Part model, mm, in its own coordinate system. A direction names the side the tool comes from. Coordinates: 2 decimals unless noted, no trailing zeros. Loops run counter-clockwise (first coordinate to the right, second up) from the corner with the lowest first, then second, coordinate; pieces in that order, holes last.
Autodesk Inventor part; units mm, degrees
ref_plane "YZ Plane" through (0, 0, 0) normal (1, 0, 0) x (0, 1, 0)
ref_plane "XZ Plane" through (0, 0, 0) normal (0, 1, 0) x (-1, 0, 0)
ref_plane "XY Plane" through (0, 0, 0) normal (0, 0, 1) x (1, 0, 0)
sketch "Sketch1" plane through (0, 0, 0) normal (0, 1, 0) x (-1, 0, 0)
  line L0 (82, 45) -> (-82, 45)
  line L1 (-90, 37) -> (-90, -37)
  line L2 (-82, -45) -> (82, -45)
  line L3 (90, -37) -> (90, 37)
  line L4 (90, 45) -> (-90, -45) construction
  line L5 (-90, 45) -> (90, -45) construction
  line L6 (90, 37) -> (82, 45)
  line L7 (90, -37) -> (82, -45)
  line L8 (-82, 45) -> (-90, 37)
  line L9 (-82, -45) -> (-90, -37)
  line L10 (90, -37) -> (80.892, -37)
  line L11 (80.892, -37) -> (80.892, -37.187)
  line L12 (80.892, -37) -> (81.079, -37) construction
  circle A0 centre (80.892, -37.187) radius 0.725
  circle A1 centre (80.892, -37.187) radius 2.225
  line L13 (90, 37) -> (80.892, 37)
  line L14 (80.892, 37) -> (80.892, 37.187)
  circle A2 centre (80.892, 37.187) radius 0.725
  circle A3 centre (80.892, 37.187) radius 2.225
  line L15 (-90, 37) -> (-80.892, 37)
  line L16 (-90, 37) -> (-80.892, 37) construction
  line L17 (-80.892, 37) -> (-80.892, 37.187)
  circle A4 centre (-80.892, 37.187) radius 0.725
  circle A5 centre (-80.892, 37.187) radius 2.225
  line L18 (-90, -37) -> (-80.892, -37)
  line L19 (-90, -37) -> (-80.892, -37) construction
  line L20 (-80.892, -37) -> (-80.892, -37.187)
  line L21 (-80.892, -37) -> (-80.705, -37) construction
  circle A6 centre (-80.892, -37.187) radius 0.725
  circle A7 centre (-80.892, -37.187) radius 2.225
  line L22 (80.892, -37.187) -> (80.892, -34.287)
  line L23 (80.892, -37.187) -> (83.792, -37.187) construction
  line L24 (80.892, -37.187) -> (77.992, -37.187)
  line L25 (80.892, -37.187) -> (83.792, -37.187) construction
  line L26 (77.992, -37.187) -> (77.992, -45)
  line L27 (80.892, 37.187) -> (80.892, 34.287)
  line L28 (80.892, 37.187) -> (83.792, 37.187) construction
  line L29 (80.892, 34.287) -> (90, 34.287)
  line L30 (80.892, 37.187) -> (77.992, 37.187)
  line L31 (80.892, 37.187) -> (83.792, 37.187) construction
  line L32 (-80.892, -37.187) -> (-80.892, -34.287)
  line L33 (-80.892, -37.187) -> (-77.992, -37.187) construction
  line L34 (-80.892, -34.287) -> (-90, -34.287)
  line L35 (-80.892, -37.187) -> (-77.992, -37.187)
  line L36 (-80.892, -37.187) -> (-77.992, -37.187) construction
  line L37 (-77.992, -37.187) -> (-77.992, -45)
  line L38 (-77.992, -37.187) -> (-70.179, -37.187) construction
  line L39 (-80.892, 37.187) -> (-77.992, 37.187)
  line L40 (-80.892, 37.187) -> (-77.992, 37.187) construction
  line L41 (-77.992, 37.187) -> (-77.992, 45)
  line L42 (-80.892, 37.187) -> (-80.892, 34.287)
  line L43 (-80.892, 37.187) -> (-77.992, 37.187) construction
  line L44 (-80.892, 34.287) -> (-90, 34.287)
  line L45 (-77.992, 37.187) -> (-77.992, 34.287)
  line L46 (-77.992, 34.287) -> (-80.892, 34.287)
  line L47 (-80.892, -34.287) -> (-77.992, -34.287)
  line L48 (-77.992, -34.287) -> (-77.992, -37.187)
  line L49 (77.992, 37.187) -> (77.992, 45)
  line L50 (77.992, 37.187) -> (85.805, 37.187) construction
  line L51 (80.892, 34.287) -> (77.992, 34.287)
  line L52 (77.992, 34.287) -> (77.992, 37.187)
  line L53 (80.892, -34.287) -> (90, -34.287)
  line L54 (80.892, -34.287) -> (90, -34.287) construction
  line L55 (77.992, -37.187) -> (77.992, -34.287)
  line L56 (77.992, -34.287) -> (80.892, -34.287)
  line L57 (-90, 0) -> (-90, 14.5)
  line L58 (-90, 0) -> (-90, -14.5)
  line L59 (-90, -14.5) -> (-86, -14.5)
  line L60 (-90, -14.5) -> (-86, -14.5) construction
  line L61 (-86, -14.5) -> (-86, 14.5)
  line L62 (-86, 14.5) -> (-90, 14.5)
  point P0 (0, 0)
  point P1 (-90, -34.287)
  point P2 (77.992, -45)
  point P3 (90, -34.287)
  point P4 (90, 34.287)
  point P5 (-90, 34.287)
  dimension "d31" = 12
  dimension "d0" = 180
  dimension "d1" = 90
  dimension "d2" = 8
  dimension "d3" = 8
  dimension "d4" = 8
  dimension "d5" = 8
  dimension "d6" = 8
  dimension "d7" = 8
  dimension "d8" = 8
  dimension "d9" = 8
  dimension "d34" = 9.108
  dimension "d35" = 0.187
  dimension "d36" = 90
  dimension "d37" = 1.45
  dimension "d38" = 4.45
  dimension "d39" = 9.108
  dimension "d40" = 0.187
  dimension "d41" = 90
  dimension "d42" = 1.45
  dimension "d43" = 4.45
  dimension "d44" = 9.108
  dimension "d45" = 0
  dimension "d46" = 0.187
  dimension "d47" = 90
  dimension "d48" = 1.45
  dimension "d49" = 4.45
  dimension "d50" = 9.108
  dimension "d51" = 0
  dimension "d52" = 0.187
  dimension "d53" = 90
  dimension "d54" = 1.45
  dimension "d55" = 4.45
  dimension "d58" = 2.9
  dimension "d59" = 90
  dimension "d62" = 2.9
  dimension "d63" = 180
  dimension "d64" = 7.813
  dimension "d65" = 90
  dimension "d66" = 2.9
  dimension "d67" = 90
  dimension "d68" = 9.108
  dimension "d69" = 90
  dimension "d70" = 2.9
  dimension "d71" = 180
  dimension "d74" = 2.9
  dimension "d75" = 90
  dimension "d76" = 9.108
  dimension "d77" = 90
  dimension "d78" = 2.9
  dimension "d79" = 0
  dimension "d80" = 7.813
  dimension "d81" = 90
  dimension "d82" = 2.9
  dimension "d83" = 0
  dimension "d84" = 7.813
  dimension "d85" = 90
  dimension "d86" = 2.9
  dimension "d87" = 90
  dimension "d88" = 9.108
  dimension "d89" = 90
  dimension "d90" = 2.9
  dimension "d91" = 2.9
  dimension "d92" = 2.9
  dimension "d93" = 2.9
extrude "Extrusion1" add sketch "Sketch1" against normal blind 2
sketch "Sketch2" plane through (0, 0, 0) normal (0, 1, 0) x (1, 0, 0)
  line L0 (-82, -45) -> (82, -45)
  line L1 (90, -37) -> (90, 37)
  line L2 (82, 45) -> (-82, 45)
  line L3 (-90, 37) -> (-90, -37)
  line L4 (-90, -45) -> (90, 45) construction
  line L5 (90, -45) -> (-90, 45) construction
  line L6 (-90, -37) -> (-82, -45)
  line L7 (-90, 37) -> (-82, 45)
  line L8 (82, 45) -> (90, 37)
  line L9 (82, -45) -> (90, -37)
  line L10 (-86, -35.3431) -> (-80.3431, -41)
  line L11 (-80.3431, -41) -> (80.3431, -41)
  line L12 (80.3431, -41) -> (86, -35.3431)
  line L13 (86, -35.3431) -> (86, 35.3431)
  line L14 (86, 35.3431) -> (80.3431, 41)
  line L15 (80.3431, 41) -> (-80.3431, 41)
  line L16 (-80.3431, 41) -> (-86, 35.3431)
  line L17 (-86, 35.3431) -> (-86, -35.3431)
  line L18 (0, 0) -> (90, 0)
  line L19 (90, 0) -> (90, -14.5)
  line L20 (90, -14.5) -> (0, -14.5)
  line L21 (0, -14.5) -> (0, 0)
  line L22 (0, 0) -> (90, 0)
  line L23 (90, 0) -> (90, 14.5)
  line L24 (90, 14.5) -> (0, 14.5)
  line L25 (0, 14.5) -> (0, 0)
  line L26 (-90, 35) -> (-81.5147, 26.5147)
  circle A0 centre (-81.5147, 26.5147) radius 1.45
  circle A1 centre (-81.5147, 26.5147) radius 4.45
  line L27 (-90, 35) -> (-77.0647, 35)
  line L28 (-77.0647, 35) -> (-77.0647, 22.0647)
  line L29 (-77.0647, 22.0647) -> (-90, 22.0647)
  line L30 (-90, 22.0647) -> (-90, 35)
  circle A2 centre (-81.5147, -26.5147) radius 1.45
  circle A3 centre (-81.5147, -26.5147) radius 4.45
  line L31 (-90, -35) -> (-77.0647, -35)
  line L32 (-77.0647, -35) -> (-77.0647, -22.0647)
  line L33 (-77.0647, -22.0647) -> (-90, -22.0647)
  line L34 (-90, -22.0647) -> (-90, -35)
  circle A4 centre (81.5147, 26.5147) radius 1.45
  circle A5 centre (81.5147, 26.5147) radius 4.45
  line L35 (77.0647, 35) -> (77.0647, 22.0647)
  line L36 (77.0647, 22.0647) -> (90, 22.0647)
  line L37 (77.0647, -22.0647) -> (90, -22.0647)
  line L38 (77.0647, -35) -> (77.0647, -22.0647)
  circle A6 centre (81.5147, -26.5147) radius 4.45
  circle A7 centre (81.5147, -26.5147) radius 1.45
  line L39 (90, -35) -> (77.0647, -35)
  line L40 (90, -22.0647) -> (90, -35)
  point P0 (86, -14.5)
  point P1 (86, 14.5)
  point P2 (81.5147, 22.0647)
  point P3 (86, 22.0647)
  point P4 (77.0647, 31)
  point P5 (77.0647, 26.5147)
  point P6 (77.0647, -26.5147)
  point P7 (77.0647, -31)
  point P8 (86, -22.0647)
  point P9 (81.5147, -22.0647)
  point P10 (-77.0647, -26.5147)
  point P11 (-81.5147, -22.0647)
  point P12 (-86, -22.0647)
  point P13 (-77.0647, -31)
  point P14 (-86, 22.0647)
  point P15 (-81.5147, 22.0647)
  point P16 (-77.0647, 26.5147)
  point P17 (-77.0647, 31)
  dimension "d12" = 180
  dimension "d13" = 90
  dimension "d14" = 8
  dimension "d15" = 8
  dimension "d16" = 8
  dimension "d17" = 8
  dimension "d18" = 8
  dimension "d19" = 8
  dimension "d20" = 8
  dimension "d21" = 8
  dimension "d22" = 4
  dimension "d23" = 90
  dimension "d24" = 14.5
  dimension "d25" = 90
  dimension "d26" = 14.5
  dimension "d31" = 12
  dimension "d32" = 2.9
  dimension "d33" = 3
extrude "Extrusion4" add sketch "Sketch2" along normal blind 10 contours L6 L3 L31 L17 L10 L11 L12 L13 L39 L1 L9 L0 | L3 L33 L17 L31 | L39 L13 L37 L1 | L3 L29 L17 L33 | L37 L13 L20 L1 | L3 L26 L17 L29 | L27 L17 L26 | L3 L7 L2 L8 L1 L36 L13 L14 L15 L16 L17 L27 | L24 L13 L36 L1
extrude "Extrusion5" add sketch "Sketch1" along normal blind 10 contours L6 L13 A3 L30 L49 L0 | L3 L29 L27 A3 L13 | L41 L39 A5 L15 L8 L0 | L30 A3 L27 L51 L52 | L45 L46 L42 A5 L39 | L3 L10 A1 L22 L53 | L15 A5 L42 L44 L1 | L7 L2 L26 L24 A1 L10 | L22 A1 L24 L55 L56 | L2 L9 L18 A7 L35 L37 | L35 A7 L32 L47 L48 | L34 L32 A7 L18 L1
extrude "Extrusion6" add sketch "Sketch1" along normal blind 8 contours L62 L61 L59 L1
fillet "Fillet1" radius 3 12 edges at (-77.992, 5, -41) (-77.992, 5, -34.287) (-86, 5, -34.287) (86, 5, -34.287) (77.992, 5, -34.287) (77.992, 5, -41) (86, 5, 34.287) (77.992, 5, 34.287) (77.992, 5, 41) (-77.992, 5, 34.287) (-86, 5, 34.287) (-77.992, 5, 41)
equation "\"d3\" = d2"
equation "\"d4\" = d2"
equation "\"d5\" = d4"
equation "\"d6\" = d2"
equation "\"d7\" = d6"
equation "\"d8\" = d2"
equation "\"d9\" = d8"
equation "\"d15\" = d14"
equation "\"d16\" = d14"
equation "\"d17\" = d16"
equation "\"d18\" = d14"
equation "\"d19\" = d18"
equation "\"d20\" = d14"
equation "\"d21\" = d20"
properties part number "enclosed base"
Q1. Drop flat-ended pins along their axis: P1, Ø0.6, axis at y = 7.5, z = -37.5, coming from the +X side; P2, Ø1.3, axis at x = 82, z = 37.5, coming from the +Y side; P3, Ø1.2, axis at x = 88, z = -0.5, coming from the +Y side. Give the stop position or say it passes through.
Q2. Saw through at C-C (y = 3.5). Count the separate pieces of the cut face and the enclosed holes in it, plus the area to 3 significant figures.
Q3. Saw through at B-B (z = 24). List the corners of the cut face in (x, y).
Q4. Tool access for faces 5 (the flat face through (1, -2, 1)), 6 (the flat face through (-86, 5, 0)): list every direction of +Z, -Z, +X, -X, +Y, -Y with a clear straight run to the whole face (end or side of a thin tool).
Q5. Probe line 1 (X direction, y = 4.75, z = 20.5); line 2 (Z direction, x = -7, y = 1.75); line 3 (Y direction, x = -34, z = 31). List the from-to ranges inside material, lowest first.
Q6. Mould opens along Z. For faces 1 (the flat face through (-1, 4, 45)), 2 (the flat face through (-86, 4, -41)), 3 (the flat face through (-90, 4, -1)), 4 (the flat face through (81, 0, -37)) say: released by +Z, released by -Z, zero draft, split by the parting line, or undercut.
Q7. Saw through at A-A (x = 41.5). List the corners of the cut face in (y, z).
Checked values:
1. P1: stops at x = 89.8
1. P2: stops at y = 0
1. P3: stops at y = 8
2. separate pieces: 1
2. enclosed holes: 5
2. area: 2,130 mm2
3. outline: (-90, -2) - (90, -2) - (90, 10) - (86, 10) - (86, 0) - (-86, 0) - (-86, 10) - (-90, 10) - close
4. face 5: +Z, -Z, +X, -X, -Y
4. face 6: +Y
5. line 1: x = -90 to -86, 86 to 90
5. line 2: z = -45 to -41, 41 to 45
5. line 3: y = -2 to 0
6. face 1: released by +Z
6. face 2: released by -Z
6. face 3: zero draft
6. face 4: undercut
7. outline: (-2, -45) - (10, -45) - (10, -41) - (0, -41) - (0, 41) - (10, 41) - (10, 45) - (-2, 45) - close
